Geometry check sheet. Reference: the model listing, model coordinates, mm. A direction names the side the tool comes from. Round coordinates to 2 decimals unless told otherwise and drop trailing zeros. Order: outer loops, then holes, each group sorted by start corner. A loop starts at its lowest first (then second) coordinate and runs counter-clockwise, first axis right, second up.
(1) Sectioned sample at B-B (x = 12.7). Record the boundary of the cut face in (y, z) (3 decimals).
(2) Sectioned sample at C-C (z = -12.7). Record the boundary of the cut face in (x, y) (3 decimals).
(3) Sectioned sample at A-A (y = 12.7). Record the boundary of the cut face in (x, z) (3 decimals).
(4) Go/stop test with flat-tipped pins: pin 1 (1.5 mm diameter, centred on x = 13.5, y = 29, fed in from -Z) (3 decimals); pin 2 (1.5 mm diameter, centred on y = 30.5, z = -8.5, fed in from +X) (3 decimals). Record where each tip stops, or that it passes through.
(5) Sectioned sample at D-D (y = 24). Record the boundary of the cut face in (x, z) (3 decimals), plus the area to 3 significant figures.
(6) Release check for a two-part mould opening along Y. For faces 3 (the face through (11.126, 14.382, -1.565)), 4 (the face through (3.175, 25, -14)), 5 (the face through (7, 0, -2)) record: +Y half, -Y half, draft (parallel to the pull), parting line (faces both ways), or undercut.
(7) Set-up check for faces 1 (the face through (14, 25, -3.175)), 2 (the face through (0, 25, -13)): record each of +Z, -Z, +X, -X, +Y, -Y from which the full face is reachable in a straight line by a thin tool's end or side.
(8) Material ranges on line 1 along Y through (x, z) = (2.2, -12.7); line 2 along Z through (x, y) = (20.25, 46) (3 decimals); line 3 along X through (y, z) = (3.5, -18) (3 decimals), recorded low to high.
from build123d import *

# Parameters (mm, degrees)
EXTRUDE_THIN1_DEPTH            = 50.8
F_9_0_196_DIAMETER_HOLE1_D     = 4.9784
F_9_0_196_DIAMETER_HOLE1_DEPTH = 3.176


with BuildPart() as part:
    # Sketch1 → Extrude-Thin1 (new body)
    with BuildSketch(Plane(origin=(0, 0, 0), x_dir=(1, 0, 0), z_dir=(0, 1, 0))):
        Polygon((25.4, 0), (0, 0), (0, 25.4), (3.175, 25.4), (3.175, 3.175), (25.4, 3.175), align=None)
    extrude(amount=EXTRUDE_THIN1_DEPTH)

    # #9 (0.196) Diameter Hole1
    with Locations(Plane(origin=(0, 0, -3.175), x_dir=(-1, 0, 0), z_dir=(0, 0, -1))):
        with Locations((-12.960193373, 12.7), (-12.7, 38.1)):
            f_9_0_196_diameter_hole1 = Hole(F_9_0_196_DIAMETER_HOLE1_D / 2, depth=F_9_0_196_DIAMETER_HOLE1_DEPTH)

    # Mirror1: #9 (0.196) Diameter Hole1 across plane
    add(f_9_0_196_diameter_hole1.mirror(Plane(origin=(0, 0, 0), x_dir=(-0.707106781, 0, 0.707106781), z_dir=(-0.707106781, 0, -0.707106781))), mode=Mode.SUBTRACT)


solid = part.part
Answer below:
1. outline: (0, -3.175) - (10.224, -3.175) - (10.224, 0) - (0, 0) - close; (15.176, -3.175) - (35.611, -3.175) - (35.611, 0) - (15.176, 0) - close; (40.589, -3.175) - (50.8, -3.175) - (50.8, 0) - (40.589, 0) - close
2. outline: (0, 0) - (3.175, 0) - (3.175, 10.224) - (0, 10.224) - close; (0, 15.176) - (3.175, 15.176) - (3.175, 35.611) - (0, 35.611) - close; (0, 40.589) - (3.175, 40.589) - (3.175, 50.8) - (0, 50.8) - close
3. outline: (0, -25.4) - (3.175, -25.4) - (3.175, -15.449) - (0, -15.449) - close; (0, -10.471) - (3.175, -10.471) - (3.175, -3.175) - (10.471, -3.175) - (10.471, 0) - (0, 0) - close; (15.449, -3.175) - (25.4, -3.175) - (25.4, 0) - (15.449, 0) - close
4. pin 1: stops at z = -3.175
4. pin 2: stops at x = 3.175
5. outline: (0, -25.4) - (3.175, -25.4) - (3.175, -3.175) - (25.4, -3.175) - (25.4, 0) - (0, 0) - close
5. area: 151 mm2
6. face 3: undercut
6. face 4: draft
6. face 5: -Y half
7. face 1: -Z, +X, +Y, -Y
7. face 2: +Z, -Z, -X, +Y, -Y
8. line 1: y = 0 to 10.22, 15.18 to 35.61, 40.59 to 50.8
8. line 2: z = -3.175 to 0
8. line 3: x = 0 to 3.175
